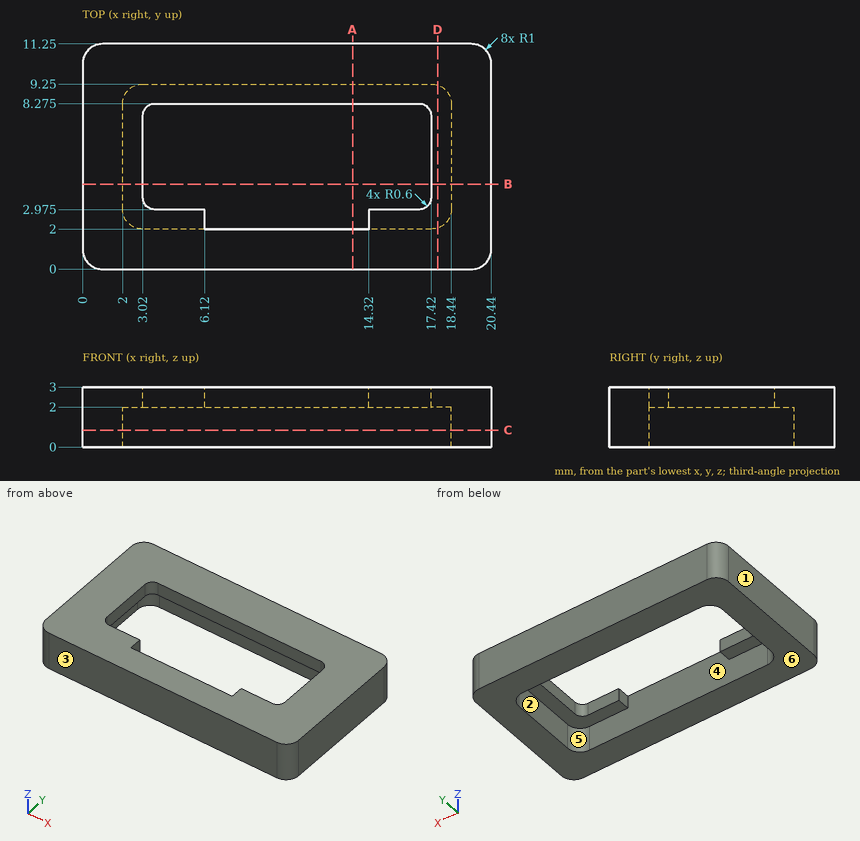
Verification items for this drawing (mm, ordinates from the low corner). A direction names the side the tool comes from. Coordinates: 2 decimals unless noted, no trailing zeros. Loops run counter-clockwise (first coordinate to the right, second up) from the corner with the lowest first, then second, coordinate; pieces in that order, holes last. Notation, with made-up numbers: (-22.75, 48.25) -> (6.25, 48.25) arc R25 cw to (6.25, 72.25) -> close; hole circle Ø2 at (-24, -15.75). An arc over 180 degrees is marked (long way). Answer in a Markdown table with one row per item. Add a question column.
1. Draft check along Y on the marked faces 3, 4, 5 and 6. Enter one of: +Y half, -Y half, draft (parallel to the pull), parting line (faces both ways), or undercut.
2. Depth check by flat-ended pin: P1, Ø0.8, axis at y = 5.5, z = 2.5, coming from the -X side; P2, Ø1, axis at x = 15.5, y = 7, coming from the -Z side. Enter the tip coordinate at first touch or a pass-through.
3. Material ranges on probe 1 along X at (y, z) = (6, 0.8); probe 2 along X at (y, z) = (6, 2.15); probe 3 along Y at (x, z) = (7.25, 1.9), recorded low to high. Write a range as [from, to].
4. Section check C-C, the plane z = 0.85. Enter the section's corners in (x, y).
5. Section check D-D, the plane x = 17.75. Enter the section's corners in (y, z), then the cut area to 3 significant figures.
6. Access from +Z, -Z, +X, -X, +Y, -Y to the whole of each face (thin tool, end or side, straight path). Record for the marked faces 1 and 2.
7. Section check A-A, the plane x = 13.5. Enter the section's corners in (y, z) (3 decimals).
8. Section check B-B, the plane y = 4.25. Enter the section's corners in (x, z), then the cut area to 3 significant figures.
Derived:
| question | item | result |
|---|---|---|
| 1 | face 3 | -Y half |
| 1 | face 4 | undercut |
| 1 | face 5 | undercut |
| 1 | face 6 | draft |
| 2 | P1 | stops at x = 0 |
| 2 | P2 | passes through |
| 3 | probe 1 | x = [0, 2], [18.44, 20.44] |
| 3 | probe 2 | x = [0, 3.02], [17.42, 20.44] |
| 3 | probe 3 | y = [0, 2], [9.25, 11.25] |
| 4 | outline | (0, 1) arc R1 ccw to (1, 0) -> (19.44, 0) arc R1 ccw to (20.44, 1) -> (20.44, 10.25) arc R1 ccw to (19.44, 11.25) -> (1, 11.25) arc R1 ccw to (0, 10.25) -> close; hole (2, 3) arc R1 ccw to (3, 2) -> (17.44, 2) arc R1 ccw to (18.44, 3) -> (18.44, 8.25) arc R1 ccw to (17.44, 9.25) -> (3, 9.25) arc R1 ccw to (2, 8.25) -> close |
| 5 | outline | (0, 0) -> (2.05, 0) -> (2.05, 2) -> (9.2, 2) -> (9.2, 0) -> (11.25, 0) -> (11.25, 3) -> (0, 3) -> close |
| 5 | area | 19.4 mm² |
| 6 | face 1 | +Z, -Z, -X, +Y, -Y |
| 6 | face 2 | -Z |
| 7 | outline | (0, 0) -> (2, 0) -> (2, 3) -> (0, 3) -> close; (8.275, 2) -> (9.25, 2) -> (9.25, 0) -> (11.25, 0) -> (11.25, 3) -> (8.275, 3) -> close |
| 8 | outline | (0, 0) -> (2, 0) -> (2, 2) -> (3.02, 2) -> (3.02, 3) -> (0, 3) -> close; (17.42, 2) -> (18.44, 2) -> (18.44, 0) -> (20.44, 0) -> (20.44, 3) -> (17.42, 3) -> close |
| 8 | area | 14.0 mm² |
